from build123d import *

# Parameters (mm, degrees)
F0_W     = 50.8
F0_H     = 38.1
F1_DEPTH = 25.4
F2_W     = 25.4
F2_H     = 12.7
F3_DEPTH = 25.4
F4_R     = 6.35
F5_DEPTH = 6.35


with BuildPart() as f1:
    # F0 (on Front) → F1 (new body)
    with BuildSketch(Plane.XZ):
        with Locations((5.782433, 3.379637)):
            Rectangle(F0_W, F0_H)
    extrude(amount=F1_DEPTH)

    # F2 (on face) → F3 (cut)
    with BuildSketch(Plane.XY.offset(22.429637)):
        with Locations((18.482433, -19.05)):
            Rectangle(F2_W, F2_H)
    extrude(amount=-F3_DEPTH, mode=Mode.SUBTRACT)

    # F4 (on face) → F5 (cut)
    with BuildSketch(Plane.XZ.offset(12.7)):
        with Locations((17.372906, 6.372478)):
            Circle(F4_R)
    extrude(amount=-F5_DEPTH, mode=Mode.SUBTRACT)


solid = f1.part
Here's how the part is built. I have some questions about the finished solid (model axes, mm). A direction names the side the tool comes from. Coordinates: 2 decimals unless noted, no trailing zeros. Write each loop counter-clockwise with the first axis right and the second up, starting at its lowest first coordinate (ties: lowest second). Pieces come first, ordered by that corner, then holes.
1) If we section it at A-A (z = -1): List the corners of the cut face in (x, y) for me, plus the area to 3 significant figures.
Filled in:
outline: (-19.62, -25.4) - (5.78, -25.4) - (5.78, -12.7) - (31.18, -12.7) - (31.18, 0) - (-19.62, 0) - close
area: 968 mm2
2) I'm going to push flat-ended pins straight in: pin 1 (7.5 mm diameter, centred on x = 21, z = 5.5, fed in from -Y); pin 2 (14 mm diameter, centred on x = 13.5, y = -21.5, fed in from +Z); pin 3 (6.5 mm diameter, centred on y = -19, z = 7.5, fed in from +X). Where does each tip first touch, or does it pass through?
Filled in:
pin 1: stops at y = -12.7
pin 2: stops at z = -2.97
pin 3: stops at x = 5.78
3) Thinking about a two-plate mould opening in X: for faces 4 (the face through (-19.618, -13, 3)), 5 (the face through (18, -12.7, 13)), 6 (the face through (17, -6.35, 6)), which applies, +X half, -X half, draft (parallel to the pull), parting line (faces both ways), or undercut?
Filled in:
face 4: -X half
face 5: draft
face 6: undercut
4) If I drill on line 1 (Z direction, x = 14, y = -21); line 2 (Y direction, x = 22, z = 3); line 3 (X direction, y = -9.75, z = 5.5), over which ranges is the centre line in solid material (lowest first)?
Filled in:
line 1: z = -15.67 to -2.97
line 2: y = -6.35 to 0
line 3: x = -19.62 to 11.08, 23.66 to 31.18
5) Which directions (+Z, -Z, +X, -X, +Y, -Y) give clear straight access to the entire face, cutting with the end or side of a thin tool? Please do faces 1 (the face through (5.782, -19, 10)), 2 (the face through (0, -10, 22.43)), 3 (the face through (23.24, -9.57, 3.94)).
Filled in:
face 1: +Z, +X, -Y
face 2: +Z, +X, -X, +Y, -Y
face 3: -Y
6) If we section it at D-D (z = 9): List the corners of the cut face in (x, y) for me, plus the area to 3 significant figures.
Filled in:
outline: (-19.62, -25.4) - (5.78, -25.4) - (5.78, -12.7) - (11.59, -12.7) - (11.59, -6.35) - (23.15, -6.35) - (23.15, -12.7) - (31.18, -12.7) - (31.18, 0) - (-19.62, 0) - close
area: 894 mm2
7) If we section it at B-B (x = 8.5): List the corners of the cut face in (y, z) for me.
Filled in:
outline: (-25.4, -15.67) - (0, -15.67) - (0, 22.43) - (-12.7, 22.43) - (-12.7, -2.97) - (-25.4, -2.97) - close
8) If we section it at C-C (y = -8.5): List the corners of the cut face in (x, z) for me, plus the area to 3 significant figures.
Filled in:
outline: (-19.62, -15.67) - (31.18, -15.67) - (31.18, 22.43) - (-19.62, 22.43) - close; hole circle Ø12.7 at (17.37, 6.37)
area: 1,810 mm2
